```python
from build123d import *

# Parameters (mm, degrees)
F2_DEPTH      = 5.08
F3_DEPTH      = 5.08
F4_DEPTH      = 2.54
F5_COUNT      = 3
F6_DEPTH      = 10.16
F7_DEPTH      = 10.16
F8_DEPTH      = 7.62
F9_DEPTH      = 2.54
F9_DEPTH_BACK = 2.54


with BuildPart() as f1:
    # F0 (on Front) → F1 (revolve)
    with BuildSketch(Plane.XZ):
        Polygon((-531.0639472567, 0), (224.2752164602, 0), (184.5656899125, 6.6608362831), (-505.6800862797, 6.6608362831), align=None)
    revolve(axis=Axis((-140.7024349097, 0, 6.6608362831), (-1, 0, 0)))

    # F0 (on Front) → F2 (join)
    with BuildSketch(Plane.XZ):
        Polygon((-503.9185357909, -16.1311917064), (-531.0639472567, 0), (-505.6800862797, 6.6608362831), (-531.0639472567, 14.332789099), (-503.9185357909, 29.4528642727), (-588.9795422554, 6.6608362831), align=None)
    extrude(amount=F2_DEPTH)

    # F0 (on Front) → F3 (join)
    with BuildSketch(Plane.XZ):
        Polygon((-503.9185357909, -16.1311917064), (-531.0639472567, 0), (-505.6800862797, 6.6608362831), (-531.0639472567, 14.332789099), (-503.9185357909, 29.4528642727), (-588.9795422554, 6.6608362831), align=None)
    extrude(amount=-F3_DEPTH)



with BuildPart() as f4:
    # F0 (on Front) → F4 (new body)
    with BuildSketch(Plane.XZ):
        Polygon((138.8282477856, 14.332789099), (177.2306859493, 14.332789099), (210.8558267355, 32.1787036955), (146.4593857527, 30.6850112975), (73.320440948, 14.332789099), align=None)
    extrude(amount=F4_DEPTH)


with BuildPart() as f5_1:
    # F5: instance of F4
    add(f4.part.rotate(Axis((-140.7024349097, 0, 6.6608362831), (-1, 0, 0)), 1 * 360 / F5_COUNT))


with BuildPart() as f5_2:
    # F5: instance of F4
    add(f4.part.rotate(Axis((-140.7024349097, 0, 6.6608362831), (-1, 0, 0)), 2 * 360 / F5_COUNT))


with BuildPart() as f1_1:
    add(f1.part)
    # F6 (add): a face of the model
    f6_faces = [f5_1.part.faces().sort_by_distance(p)[0] for p in [
        (125.2755634487, 7.2791060352, 3.924712138),
    ]]

    add(f5_1.part)  # F6 merges F5_1
    extrude(f6_faces, amount=F6_DEPTH)

    # F7 (add): a face of the model
    f7_faces = [f4.part.faces().sort_by_distance(p)[0] for p in [
        (125.2755634487, -1.27, 14.332789099),
    ]]

    add(f4.part)  # F7 merges F4
    extrude(f7_faces, amount=F7_DEPTH)

    # F8 (add): a face of the model
    f8_faces = [f5_2.part.faces().sort_by_distance(p)[0] for p in [
        (125.2755634487, -6.0091060352, 1.7250076124),
    ]]

    add(f5_2.part)  # F8 merges F5_2
    extrude(f8_faces, amount=F8_DEPTH)

    # F0 (on Front) → F9 (join, two sides)
    with BuildSketch(Plane.XZ) as f9_sk:
        Polygon((184.5656899125, 6.6608362831), (224.2752164602, 6.6608362831), (230.9360527433, 14.332789099), (177.2306859493, 14.332789099), (138.8282477856, 14.332789099), align=None)
        Polygon((224.2752164602, 0), (231.9471692761, 0), (224.2752164602, 6.6608362831), (184.5656899125, 6.6608362831), align=None)
    extrude(amount=F9_DEPTH)
    extrude(f9_sk.sketch, amount=-F9_DEPTH_BACK)


solid = f1_1.part
```
CAD build for the part. Positions are in the model's coordinates, mm. A direction names the side the tool comes from. Coordinates: 2 decimals unless noted, no trailing zeros. Order: outer loops, then holes, each group sorted by start corner. A loop starts at its lowest first (then second) coordinate and runs counter-clockwise, first axis right, second up. Notation, with made-up numbers: (52.25, 17.5) - (87.25, 17.5) arc R13 ccw to (87.25, 41.5) - close; hole circle Ø9 at (28, -6.75). An arc over 180 degrees is marked (long way). Use a Markdown table: item, result. Add a question column.
(1) Which spindle directions (+Z, -Z, +X, -X, +Y, -Y) get a long thin tool onto all of the face, cutting with end or side? Do faces 4 (the face through (-148.107, -2.001, 0.308)), 5 (the face through (156.41, 12.23, -0.4)), 6 (the face through (110.402, 14.45, -0.236)), 7 (the face through (110.402, -1.252, 22.623)). Say none if no direction does.
(2) Saw through at A-A (x = 40). Give the cut face in (y, z), then the cut area to 3 significant figures.
(3) Pull direction Z, two halves, no side cores. Call faces 1 (the face through (-545.854, -0.071, 18.216)), 2 (the face through (-547.044, -0.071, -4.576)), 3 (the face through (-517.681, -0.071, 21.787)): +Z half, -Z half, draft (parallel to the pull), parting line (faces both ways), or undercut.
(4) Flat gauge pins, fed straight in: pin 1 (12 mm diameter, centred on x = -88, y = 0, fed in from -Z); pin 2 (3 mm diameter, centred on y = -5, z = 2.5, fed in from +X); pin 3 (4 mm diameter, centred on x = -200.5, y = 8, fed in from -Z); pin 4 (1 mm diameter, centred on x = -131, y = 7.5, fed in from +Z). Where does each tip first touch, or does it go through?
(5) Drill centre lines: line 1 along Z through (x, y) = (4, -5); line 2 along Z through (x, y) = (6, -1); line 3 along Y through (x, z) = (-79.5, 3.5). Where is each one in solid material? Low to high. Write a range as [from, to].
Solved:
| question | item | result |
|---|---|---|
| 1 | face 4 | none |
| 1 | face 5 | -Z, +X, -X |
| 1 | face 6 | -Z, -X, +Y |
| 1 | face 7 | +Z, +Y, -Y |
| 2 | outline | circle Ø13.32 at (0, 6.66) |
| 2 | area | 139 mm² |
| 3 | face 1 | +Z half |
| 3 | face 2 | -Z half |
| 3 | face 3 | undercut |
| 4 | pin 1 | stops at z = 0 |
| 4 | pin 2 | stops at x = 224.28 |
| 4 | pin 3 | stops at z = 3.77 |
| 4 | pin 4 | passes through |
| 5 | line 1 | z = [2.26, 11.06] |
| 5 | line 2 | z = [0.08, 13.25] |
| 5 | line 3 | y = [-5.86, 5.86] |
